Can you work these out from the model? Positions are in its coordinate system, mm. A direction names the side the tool comes from. Give positions to 0.01 mm unless a question says otherwise; leave off trailing zeros. Order: outer loops, then holes, each group sorted by start corner. A loop starts at its lowest first (then second) coordinate and runs counter-clockwise, first axis right, second up. Notation, with made-up numbers: (-14, 1.5) - (6, 1.5) arc R24 cw to (6, 17.5) - close; hole circle Ø10 at (-2.5, 23). An arc over 180 degrees is marked (long way). One line per question, with ' | ' between items.
```python
from build123d import *

# Parameters (mm, degrees)
SKETCH1_W           = 340.2
SKETCH1_H           = 20
BOSS_EXTRUDE1_DEPTH = 20
FILLET1_R           = 2
CUT_EXTRUDE1_DEPTH  = 21
SKETCH3_W           = 16
SKETCH3_H           = 16
CUT_EXTRUDE2_DEPTH  = 611.1


with BuildPart() as part:
    # Sketch1 → Boss-Extrude1 (new body)
    with BuildSketch(Plane.XY):
        with Locations((-440, -1090)):
            Rectangle(SKETCH1_W, SKETCH1_H)
    extrude(amount=-BOSS_EXTRUDE1_DEPTH)

    # Fillet1
    fillet1_edges = [part.edges().sort_by_distance(p)[0] for p in [
        (-440, -1100, -20),
        (-440, -1100, 0),
        (-440, -1080, 0),
        (-440, -1080, -20),
    ]]
    fillet(fillet1_edges, radius=FILLET1_R)

    # Sketch2 → Cut-Extrude1 (cut, through all)
    with BuildSketch(Plane.XY):
        Polygon((-269.9, -1100), (-269.9, -1080), (-289.9, -1080), align=None)
        Polygon((-610.1, -1100), (-590.1, -1080), (-610.1, -1080), align=None)
    extrude(amount=-CUT_EXTRUDE1_DEPTH, mode=Mode.SUBTRACT)

    # Sketch3 → Cut-Extrude2 (cut, through all)
    with BuildSketch(Plane(origin=(0, 0, 0), x_dir=(0, 0, -1), z_dir=(1, 0, 0))):
        with Locations((10, -1090)):
            Rectangle(SKETCH3_W, SKETCH3_H)
    extrude(amount=-CUT_EXTRUDE2_DEPTH, mode=Mode.SUBTRACT)


solid = part.part
```
(1) If we mould it in two halves opening along Y, with no side actions, what happens to faces 1 (the face through (-442, -1080, -10)), 2 (the face through (-438, -1098, -10)), 3 (the face through (-442, -1100, -10))? For each: released by +Y, released by -Y, zero draft, split by the parting line, or undercut.
Answer below:
face 1: released by +Y | face 2: undercut | face 3: released by -Y
(2) Imagine slicing it at A-A (y = -1089.75). List the corners of the cut face in (x, z) for me.
Answer below:
outline: (-599.85, -20) - (-280.15, -20) - (-280.15, -18) - (-599.85, -18) - close; (-599.85, -2) - (-280.15, -2) - (-280.15, 0) - (-599.85, 0) - close
(3) On a 3-axis mill with a long thin cutter (end or side, diameter ignored), from which of +Z, -Z, +X, -X, +Y, -Y can I reach the whole of each face in a straight line? I mean faces 4 (the face through (-438, -1082, -10)), 5 (the face through (-442, -1090, 0)). Say none if no direction works.
Answer below:
face 4: +X, -X | face 5: +Z, +X, -X, +Y, -Y
(4) If I drill on line 1 (Y direction, x = -401.5, z = -14.5); line 2 (Z direction, x = -514, y = -1091); line 3 (Y direction, x = -285, z = -11.75), over which ranges is the centre line in solid material (lowest first)?
Answer below:
line 1: -1100 to -1098, -1082 to -1080 | line 2: -20 to -18, -2 to 0 | line 3: -1100 to -1098
(5) Imagine slicing it at C-C (x = -401.5). List the corners of the cut face in (y, z) for me, and give its area (3 significant figures).
Answer below:
outline: (-1100, -18) arc R2 ccw to (-1098, -20) - (-1082, -20) arc R2 ccw to (-1080, -18) - (-1080, -2) arc R2 ccw to (-1082, 0) - (-1098, 0) arc R2 ccw to (-1100, -2) - close; hole (-1098, -18) - (-1082, -18) - (-1082, -2) - (-1098, -2) - close | area: 141 mm^2
(6) Will this pin go through, and if not, where does the flat tip stop? pin 1 (10 mm diameter, centred on y = -1083.5, z = -13.5, fed in from +X).
Answer below:
pin 1: x = -284.22
(7) Imagine slicing it at B-B (z = -7.75). List the corners of the cut face in (x, y) for me.
Answer below:
outline: (-610.1, -1100) - (-269.9, -1100) - (-271.9, -1098) - (-608.1, -1098) - close; (-592.1, -1082) - (-287.9, -1082) - (-289.9, -1080) - (-590.1, -1080) - close
